Could you check a few things on this model? Use its own coordinates, in mm. A direction names the side the tool comes from. Coordinates: 2 decimals unless noted, no trailing zeros. Answer as a JSON object with one key per item and string values. Group by question number.
(1) We'd pull the mould along Y, two halves only. Please class faces 1 (the cylindrical face through (16.32, 72.72, 6.86)), 2 (the flat face through (20, 68, -7)), 3 (the flat face through (33.88, 68.67, 0.15)): pulls with the +Y half, pulls with the -Y half, needs draft (parallel to the pull), parting line crosses it, or undercut.
(2) Will these pins go through, and if not, where does the flat tip stop? P1, Ø8, axis at y = 70, z = 11.5, coming from the -X side; P2, Ø5, axis at x = 16.5, y = 70.5, coming from the -Z side; P3, Ø2, axis at x = 28, y = 74.5, coming from the +Z side.
(3) Imagine slicing it at A-A, the plane x = 15. Give the number of separate pieces and of enclosed holes in the cut face, and give its area (3 significant figures).
(4) Please list where these lines run through material, in increasing order: probe 1 along Z at (x, y) = (22, 67.5); probe 2 along X at (y, z) = (65, 2.75); probe 3 along X at (y, z) = (63, 6).
(5) Which directions (+Z, -Z, +X, -X, +Y, -Y) give clear straight access to the entire face, cutting with the end or side of a thin tool? Please do faces 4 (the flat face through (25.2, 64.88, -0.09)), 5 (the conical face through (14.41, 82.67, -0.46)), 6 (the flat face through (19.487, 77.284, 0.091)).
from build123d import *

# Parameters (mm, degrees)
BOSS_EXTRUDE1_DEPTH      = 7
BOSS_EXTRUDE1_DEPTH_BACK = 7
SKETCH2_R                = 3.0000000000000018
BOSS_EXTRUDE2_DEPTH      = 2
BOSS_EXTRUDE2_DEPTH_BACK = 2
SKETCH3_R                = 14.700000000000001
BOSS_EXTRUDE3_START      = 5
SKETCH4_R                = 14.700000000000001
SKETCH4_R_2              = 12.699999999999998
BOSS_EXTRUDE3_DEPTH      = 5
FILLET2_R                = 0.5
FILLET4_R                = 0.5
CHAMFER1_SIZE            = 0.5
CHAMFER2_SIZE            = 1
CUT_EXTRUDE1_DEPTH       = 54.24291481918433


with BuildPart() as part:
    # Sketch2 → Boss-Extrude1 (new, two sides: drawn at the far end of the back side and taken through both)
    with BuildSketch(Plane.XY.offset(-BOSS_EXTRUDE1_DEPTH_BACK)):
        with BuildLine():
            Line((30.512377936980783, 70.89647327651264), (21.781878923827843, 61.0053372557492))
            ThreePointArc((21.781878923827843, 61.0053372557492), (13.313031061350836, 60.477496482202135), (12.78519028780376, 68.94634434467913))
            Line((12.78519028780376, 68.94634434467913), (21.51568930095671, 78.83748036544256))
            Line((21.51568930095671, 78.83748036544256), (30.512377936980783, 70.89647327651264))
        make_face()
        with Locations((17.283534605815802, 64.97584080021417)):
            Circle(SKETCH2_R, mode=Mode.SUBTRACT)
    extrude(amount=BOSS_EXTRUDE1_DEPTH + BOSS_EXTRUDE1_DEPTH_BACK)

    # Sketch3 → Boss-Extrude2 (add, two sides: drawn at the far end of the back side and taken through both)
    with BuildSketch(Plane(origin=(48.53568375746082, 54.98804239970119, 0), x_dir=(0.7497240530020064, -0.66175059074416, 0), z_dir=(0.66175059074416, 0.7497240530020064, 0)).offset(-BOSS_EXTRUDE2_DEPTH_BACK)):
        with Locations(Location((-30.039919418767553, 0, 0), (0, 0, 180))):
            Circle(SKETCH3_R)
    extrude(amount=BOSS_EXTRUDE2_DEPTH + BOSS_EXTRUDE2_DEPTH_BACK)

    # Sketch4 → Boss-Extrude3 (add)
    with BuildSketch(Plane(origin=(49.85918493894915, 56.48749050570521, 0), x_dir=(0.7497240530020064, -0.66175059074416, 0), z_dir=(0.66175059074416, 0.7497240530020064, 0)).offset(BOSS_EXTRUDE3_START)):
        with Locations(Location((-30.03991941876756, 0, 0), (0, 0, 180))):
            Circle(SKETCH4_R)
        with Locations(Location((-30.03991941876756, 0, 0), (0, 0, 180))):
            Circle(SKETCH4_R_2, mode=Mode.SUBTRACT)
    extrude(amount=-BOSS_EXTRUDE3_DEPTH)

    # Fillet2
    fillet2_edges = [part.edges().sort_by_distance(p)[0] for p in [
        (41.66723133330735, 70.38731150805249, 3.6e-15),
        (40.16778322730333, 71.7108126895408, 3.11e-15),
    ]]
    fillet(fillet2_edges, radius=FILLET2_R)

    # Fillet4
    fillet4_edges = [part.edges().sort_by_distance(p)[0] for p in [
        (13.313031061350841, 60.47749648220213, 7),
        (25.48537783966015, 65.2011812131289, 7),
        (16.488689203636067, 73.14218830205883, 7),
        (25.48537783966015, 65.2011812131289, -7),
        (16.488689203636067, 73.14218830205883, -7),
        (13.313031061350841, 60.47749648220213, -7),
    ]]
    fillet(fillet4_edges, radius=FILLET4_R)

    # Chamfer1
    chamfer1_edges = [part.edges().sort_by_distance(p)[0] for p in [
        (14.2835346058158, 64.97584080021417, -7),
        (14.2835346058158, 64.97584080021417, 7),
    ]]
    chamfer(chamfer1_edges, length=CHAMFER1_SIZE)

    # Chamfer2
    chamfer2_edges = [part.edges().sort_by_distance(p)[0] for p in [
        (35.711476016609915, 63.639795031034424, 3.6e-15),
        (24.690532437480417, 73.36752871497357, -7),
        (29.188876755492455, 69.39702517050861, -2.2e-16),
        (20.192188119468376, 77.33803225943853, -2.2e-16),
        (24.690532437480417, 73.36752871497357, 7),
        (29.079082209939642, 69.493936300796, -6.853553390593275),
        (20.301982665021182, 77.24112112915115, -6.853553390593271),
        (29.079082209939642, 69.493936300796, 6.853553390593275),
        (20.301982665021182, 77.24112112915115, 6.853553390593271),
    ]]
    chamfer(chamfer2_edges, length=CHAMFER2_SIZE)

    # Sketch5 → Cut-Extrude1 (cut, through all)
    with BuildSketch(Plane(origin=(53.16793789266995, 60.23611077071524, 0), x_dir=(0.7497240530020064, -0.66175059074416, 0), z_dir=(0.66175059074416, 0.7497240530020064, 0))):
        Polygon((-10.039919418767552, 12.5), (-10.039919418767552, -12.5), (-20.03991941876755, -12.500000000000004), (-20.03991941876755, 12.500000000000004), align=None)
    extrude(amount=-CUT_EXTRUDE1_DEPTH, mode=Mode.SUBTRACT)


solid = part.part
Result set:
{
 "1": {"face 1": "undercut", "face 2": "needs draft", "face 3": "pulls with the -Y half"},
 "2": {"P1": "stops at x = 23.97", "P2": "stops at z = -7", "P3": "stops at z = 14.68"},
 "3": {"separate pieces": "3", "enclosed holes": "0", "area": "135 mm^2"},
 "4": {"probe 1": "z = -7 to 7", "probe 2": "x = 11.28 to 14.28, 20.28 to 25.31", "probe 3": "x = 11.62 to 15.03, 19.54 to 23.54"},
 "5": {"face 4": "+Z, -Z, -Y", "face 5": "-X", "face 6": "+Z, -Z, -X"}
}
